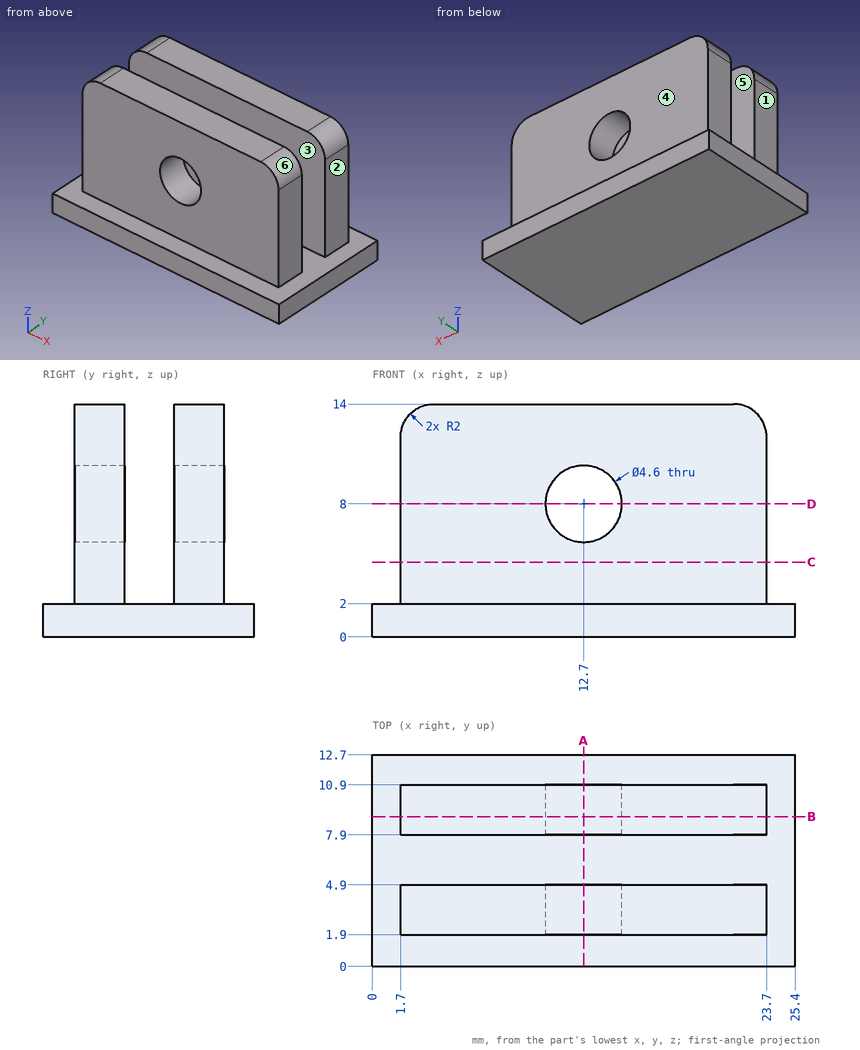
Input: dimensioned drawing with shaded views. Units: mm. Origin: part minimum x, y, z. A direction names the side the tool comes from. Coordinates: 2 decimals unless noted, no trailing zeros. Write each loop counter-clockwise with the first axis right and the second up, starting at its lowest first coordinate (ties: lowest second). Pieces come first, ordered by that corner, then holes. Notation, with made-up numbers: M -21,18.5 L 30,18.5 A33 cw 30,51.5 Z; hole C 0,88 d10. An arc over 180 degrees is marked long. Use one line per item in the form item = value.
Q1. Section D-D (z = 8). Return loops of the section in (x, y).
Answer below:
outline = M 1.7,1.9 L 10.4,1.9 L 10.4,4.9 L 1.7,4.9 Z; M 1.7,7.9 L 10.4,7.9 L 10.4,10.9 L 1.7,10.9 Z; M 15,1.9 L 23.7,1.9 L 23.7,4.9 L 15,4.9 Z; M 15,7.9 L 23.7,7.9 L 23.7,10.9 L 15,10.9 Z
Q2. Material intervals for probe 1 along Y at (x, z) = (14.75, 11); probe 2 along Z at (x, y) = (12.7, 9.8); probe 3 along Z at (x, y) = (16.75, 11), sorted ascending. Write a range as from..to.
Answer below:
probe_1 = 1.9..4.9, 7.9..10.9
probe_2 = 0..5.7, 10.3..14
probe_3 = 0..2
Q3. First-contact query: pin 1 (0.9 mm diameter, centred on y = 2.5, z = 5, fed in from -X); pin 2 (5 mm diameter, centred on x = 7.5, z = 6, fed in from -Y); pin 3 (3.5 mm diameter, centred on y = 3, z = 5.5, fed in from +X); pin 4 (8 mm diameter, centred on x = 18, z = 5, fed in from +Y). Flat tips, straight axial feed; report the tip coordinate or a pass-through.
Answer below:
pin_1 = 1.7
pin_2 = 1.9
pin_3 = 23.7
pin_4 = 12.7
Q4. Draft query along Y for the marked faces 4, 5 and 6. Return one class per face: released by +Y, released by -Y, zero draft, split by the parting line, or undercut.
Answer below:
face_4 = released by +Y
face_5 = undercut
face_6 = zero draft
Q5. Set-up query: the marked faces 1, 2 and 3. Return all of +Z, -Z, +X, -X, +Y, -Y with unobstructed straight access to the full face (end or side cutting, diameter ignored); none if empty.
Answer below:
face_1 = +Z, -X, +Y, -Y
face_2 = +Z, +X, +Y, -Y
face_3 = +Z, +X, -X
Q6. Section B-B (y = 9). Return loops of the section in (x, z).
Answer below:
outline = M 0,0 L 25.4,0 L 25.4,2 L 23.7,2 L 23.7,12 A2 ccw 21.7,14 L 3.7,14 A2 ccw 1.7,12 L 1.7,2 L 0,2 Z; hole C 12.7,8 d4.6
Q7. Section C-C (z = 4.5). Return loops of the section in (x, y), plus the area to 3 significant figures.
Answer below:
outline = M 1.7,1.9 L 23.7,1.9 L 23.7,4.9 L 1.7,4.9 Z; M 1.7,7.9 L 23.7,7.9 L 23.7,10.9 L 1.7,10.9 Z
area = 132 mm²
Q8. Section A-A (x = 12.7). Return loops of the section in (y, z), plus the area to 3 significant figures.
Answer below:
outline = M 0,0 L 12.7,0 L 12.7,2 L 10.9,2 L 10.9,5.7 L 7.9,5.7 L 7.9,2 L 4.9,2 L 4.9,5.7 L 1.9,5.7 L 1.9,2 L 0,2 Z; M 1.9,10.3 L 4.9,10.3 L 4.9,14 L 1.9,14 Z; M 7.9,10.3 L 10.9,10.3 L 10.9,14 L 7.9,14 Z
area = 69.8 mm²
